from build123d import *

# Parameters (mm, degrees)
ESBO_O1_R                  = 1.5
RESSALTO_EXTRUS_O1_DEPTH   = 30
FILETE1_R                  = 5
CORTE_EXTRUS_O1_DEPTH      = 37.349002737
CORTE_EXTRUS_O1_DEPTH_BACK = 37.349002737
ESBO_O2_R                  = 1.5
ESBO_O2_W                  = 10.5
ESBO_O2_H                  = 10.5


with BuildPart() as part:
    # Esboço1 → Ressalto-extrusão1 (new body)
    with BuildSketch(Plane.XY):
        with BuildLine():
            Line((-9, 0), (9, 0))
            Line((9, 0), (9, -2.5))
            Line((9, -2.5), (-14.585891007, -2.5))
            Line((-14.585891007, -2.5), (-16.925971737, 7.837663684))
            ThreePointArc((-16.925971737, 7.837663684), (-14.662336316, 11.425971737), (-11.074028263, 9.162336316))
            Line((-11.074028263, 9.162336316), (-9, 0))
        make_face()
        with Locations((-14, 8.5)):
            Circle(ESBO_O1_R, mode=Mode.SUBTRACT)
    extrude(amount=RESSALTO_EXTRUS_O1_DEPTH)

    # Filete1
    filete1_edges = [part.edges().sort_by_distance(p)[0] for p in [
        (-14.585891007, -2.5, 15),
        (-9, 0, 15),
    ]]
    fillet(filete1_edges, radius=FILETE1_R)

    # Esboço2 → Corte-extrusão1 (cut, two sides: drawn at the far end of the back side and taken through both)
    with BuildSketch(Plane(origin=(0, 0, 0), x_dir=(1, 0, 0), z_dir=(0, 1, 0)).offset(-CORTE_EXTRUS_O1_DEPTH_BACK)):
        with Locations(Location((0, -7, 0), (0, 0, 180))):
            Circle(ESBO_O2_R)
        with Locations(Location((0, -23, 0), (0, 0, 180))):
            Circle(ESBO_O2_R)
        with Locations((-11.75, -8.25)):
            Rectangle(ESBO_O2_W, ESBO_O2_H)
        with Locations((-11.75, -21.75)):
            Rectangle(ESBO_O2_W, ESBO_O2_H)
    extrude(amount=CORTE_EXTRUS_O1_DEPTH + CORTE_EXTRUS_O1_DEPTH_BACK, mode=Mode.SUBTRACT)


solid = part.part
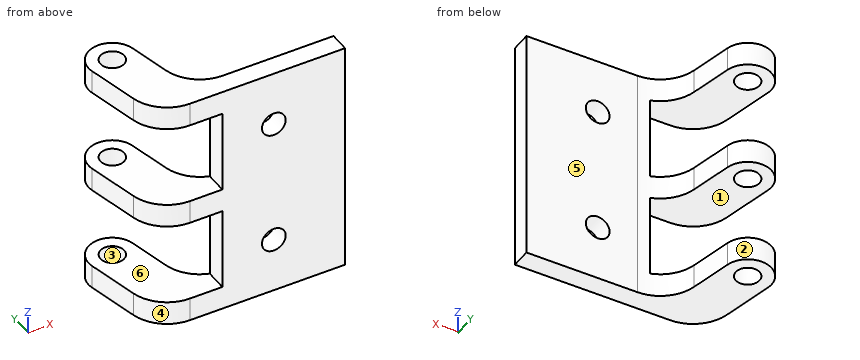
Source: CAD feature listing. Evaluate the final solid. Frame: model axes, mm. Face numbers are marked on the shaded views. A direction names the side the tool comes from. Give positions to 0.01 mm unless a question says otherwise; leave off trailing zeros. Order: outer loops, then holes, each group sorted by start corner. A loop starts at its lowest first (then second) coordinate and runs counter-clockwise, first axis right, second up. Notation, with made-up numbers: (-21.5, 29.25) -> (17.5, 29.25) arc R28 cw to (17.5, 66.25) -> close; hole circle Ø8 at (-15, 68.5). An arc over 180 degrees is marked (long way). Use a Markdown table: item, result.
1) Section query B-B, the plane x = 0. Return the cut outline in (y, z), then the cut area to 3 significant figures.
Answer list:
| item | result |
|---|---|
| outline | (-2.5, 0) -> (0, 0) -> (0, 5.5) -> (-2.5, 5.5) -> close; (-2.5, 8.5) -> (0, 8.5) -> (0, 21.5) -> (-2.5, 21.5) -> close; (-2.5, 24.5) -> (0, 24.5) -> (0, 30) -> (-2.5, 30) -> close |
| area | 60.0 mm² |
2) Ray query, line 1 along Z through (x, y) = (-9, 0.25); line 2 along Z through (x, y) = (0, -1.95); line 3 along X through (y, z) = (-1.75, 23). Return the intervals inside material, ascending. Write a range as [from, to].
Answer list:
| item | result |
|---|---|
| line 1 | [0, 3], [13.5, 16.5], [27, 30] |
| line 2 | [0, 5.5], [8.5, 21.5], [24.5, 30] |
| line 3 | [-6.5, -1.5], [1.5, 9] |
3) Section query C-C, the plane y = 5. Return the cut outline in (x, z), then the cut area to 3 significant figures.
Answer list:
| item | result |
|---|---|
| outline | (-16.28, 0) -> (-10.13, 0) -> (-10.13, 3) -> (-16.28, 3) -> close; (-16.28, 13.5) -> (-10.13, 13.5) -> (-10.13, 16.5) -> (-16.28, 16.5) -> close; (-16.28, 27) -> (-10.13, 27) -> (-10.13, 30) -> (-16.28, 30) -> close |
| area | 55.4 mm² |
4) Section query D-D, the plane z = 7. Return the cut outline in (x, y).
Answer list:
| item | result |
|---|---|
| outline | (-6.5, -2.5) -> (-1.5, -2.5) -> (-1.5, 0) -> (-5.01, 0) arc R5 cw to (-6.5, 0.23) -> close; (1.5, -2.5) -> (9, -2.5) -> (9, 0) -> (1.5, 0) -> close |
5) Section query A-A, the plane z = 27.5. Return the cut outline in (x, y).
Answer list:
| item | result |
|---|---|
| outline | (-16.93, 7.84) -> (-15.47, 1.4) arc R5 ccw to (-10.59, -2.5) -> (9, -2.5) -> (9, 0) -> (-5.01, 0) arc R5 cw to (-9.88, 3.9) -> (-11.07, 9.16) arc R3 ccw to start; hole circle Ø3 at (-14, 8.5) |
6) Contact query for flat-ended pins moving along their axis: P1, Ø2, axis at y = -1, z = 7.5, coming from the -X side; P2, Ø7, axis at x = 2, z = 17.5, coming from the +Y side. Output: stop coordinate, or through.
Answer list:
| item | result |
|---|---|
| P1 | x = -6.5 |
| P2 | y = 0 |
7) Reachability of the marked faces 4, 5 and 6 from +Z, -Z, +X, -X, +Y, -Y: full face, straight path, thin tool, end or side. Return the list, or none.
Answer list:
| item | result |
|---|---|
| face 4 | +Z, -Z, -X, -Y |
| face 5 | +Z, -Z, +X, +Y |
| face 6 | -X, +Y, -Y |
8) Mould query, pull axis X, two halves, no side actions, for the marked faces 1, 2 and 3. Classes: +X half, -X half, draft (parallel to the pull), parting line (faces both ways), or undercut.
Answer list:
| item | result |
|---|---|
| face 1 | draft |
| face 2 | parting line |
| face 3 | undercut |
